Source: CAD feature listing. Evaluate the final solid. Frame: model axes, mm. Face numbers are marked on the shaded views. Give positions to 0.01 mm unless a question says otherwise; leave off trailing zeros. Write each loop counter-clockwise with the first axis right and the second up, starting at its lowest first coordinate (ties: lowest second). Pieces come first, ordered by that corner, then holes. Notation, with made-up numbers: M 41.25,68 L 83.25,68 A23 ccw 83.25,86 Z; hole C 40.5,31 d11. An arc over 180 degrees is marked long. Return JSON: item names as keys, results as strings.
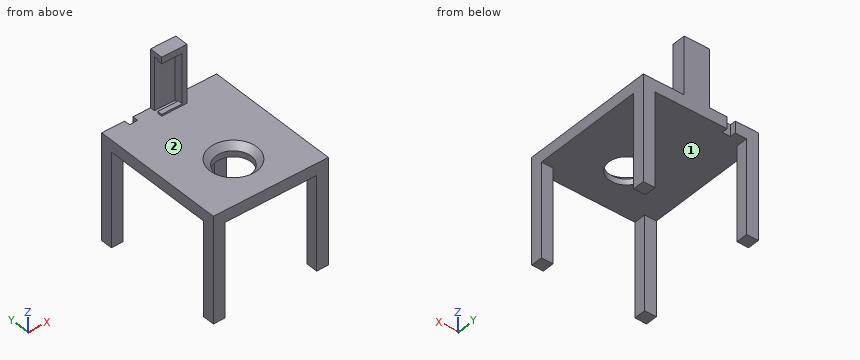
Autodesk Inventor part; units mm, degrees
ref_plane "YZ Plane" through (0, 0, 0) normal (1, 0, 0) x (0, 1, 0)
ref_plane "XZ Plane" through (0, 0, 0) normal (0, 1, 0) x (-1, 0, 0)
ref_plane "XY Plane" through (0, 0, 0) normal (0, 0, 1) x (1, 0, 0)
sketch "Skizze1" plane through (0, 0, 0) normal (0, 0, 1) x (1, 0, 0)
  line L0 (-19.6, 0) -> (117.6, 0)
  line L1 (0, -23) -> (0, 138)
  line L2 (0, 0) -> (98, 0)
  line L3 (98, 0) -> (98, 115)
  line L4 (98, 115) -> (0, 115)
  line L5 (0, 115) -> (0, 0)
  point P0 (0, 115)
  dimension "d0" = 115
  dimension "d1" = 98
extrude "Extrusion1" add sketch "Skizze1" along normal blind 10
sketch "Skizze2" plane through (0, 0, 10) normal (0, 0, 1) x (1, 0, 0)
  line L0 (98, 115) -> (0, 115)
  line L1 (41.65, 115) -> (63.15, 115)
  line L2 (63.15, 115) -> (63.15, 103.5)
  line L3 (63.15, 103.5) -> (41.65, 103.5)
  line L4 (41.65, 103.5) -> (41.65, 115)
  line L5 (98, 0) -> (98, 115)
  point P0 (0, 0)
  dimension "d4" = 21.5
  dimension "d5" = 11.5
  dimension "d6" = 34.85
extrude "Extrusion2" add sketch "Skizze2" along normal blind 49.2
sketch "Skizze3" plane through (41.65, 103.5, 10) normal (-1, 0, 0) x (0, 0, 1)
  line L0 (45.2, 7.5) -> (45.2, 4)
  line L1 (45.2, 4) -> (43.7, 4)
  line L2 (43.7, 4) -> (43.7, 2.8888)
  line L3 (0, 0) -> (0, 11.5)
  line L4 (45.2, 7.5) -> (0, 7.5)
  line L5 (0, 11.5) -> (0, 0)
  line L6 (0, 4) -> (0, 7.5)
  line L7 (49.2, 11.5) -> (49.2, 0)
  line L8 (0, 11.5) -> (49.2, 11.5)
  line L9 (0, 0) -> (49.2, 0)
  line L10 (1.5, 2.8888) -> (1.5, 4)
  line L11 (1.5, 4) -> (0, 4)
  line L12 (43.7, 2.8888) -> (43.7, 0)
  line L13 (1.5, 2.8888) -> (1.5, 0)
  point P0 (-10, -103.5)
  point P1 (0, 4)
  dimension "d9" = 4
  dimension "d10" = 4
  dimension "d11" = 4
  dimension "d12" = 4
  dimension "d13" = 1.5
  dimension "d14" = 1.5
extrude "Extrusion3" cut sketch "Skizze3" against normal blind 17.5 contours L0 L1 L2 L12 L9 L13 L10 L11 L3 L4
sketch "Skizze4" plane through (0, 0, 10) normal (0, 0, 1) x (1, 0, 0)
  line L0 (98, 115) -> (0, 115)
  line L1 (19.65, 115) -> (26.65, 115)
  line L2 (26.65, 115) -> (26.65, 110)
  line L3 (26.65, 110) -> (19.65, 110)
  line L4 (19.65, 110) -> (19.65, 115)
  line L5 (41.65, 115) -> (41.65, 103.5)
  point P0 (0, 0)
  dimension "d17" = 7
  dimension "d18" = 5
  dimension "d19" = 15
extrude "Extrusion4" cut sketch "Skizze4" against normal blind 10
sketch "Skizze5" plane through (0, 0, 0) normal (0, 0, -1) x (-1, 0, 0)
  line L0 (-19.65, 115) -> (0, 115)
  line L1 (0, 115) -> (0, 0)
  line L2 (-10, 115) -> (0, 115)
  line L3 (0, 115) -> (0, 105)
  line L4 (0, 105) -> (-10, 105)
  line L5 (-10, 105) -> (-10, 115)
  line L6 (0, 0) -> (-98, 0)
  line L7 (0, 10) -> (-10, 10)
  line L8 (-10, 10) -> (-10, 0)
  line L9 (-10, 0) -> (0, 0)
  line L10 (0, 0) -> (0, 10)
  line L11 (-98, 10) -> (-88, 10)
  line L12 (-88, 10) -> (-88, 0)
  line L13 (-88, 0) -> (-98, 0)
  line L14 (-98, 0) -> (-98, 10)
  line L15 (-98, 115) -> (-26.65, 115)
  line L16 (-88, 115) -> (-98, 115)
  line L17 (-98, 115) -> (-98, 105)
  line L18 (-98, 105) -> (-88, 105)
  line L19 (-88, 105) -> (-88, 115)
  line L20 (-98, 0) -> (-98, 115)
  point P0 (-98, 0)
  point P1 (-88, 0)
  dimension "d22" = 10
  dimension "d23" = 10
  dimension "d24" = 10
  dimension "d25" = 10
  dimension "d26" = 10
  dimension "d27" = 10
  dimension "d28" = 10
  dimension "d29" = 10
  dimension "d40" = 0
extrude "Extrusion5" add sketch "Skizze5" along normal blind 80
sketch "Skizze6" plane through (0, 0, 10) normal (0, 0, 1) x (1, 0, 0)
  circle A0 centre (49, 38.5) radius 15
  line L0 (0, 115) -> (0, 0)
  line L1 (41.65, 103.5) -> (63.15, 103.5)
  dimension "d32" = 30
  dimension "d33" = 49
  dimension "d34" = 65
extrude "Extrusion6" cut sketch "Skizze6" against normal blind 10
chamfer "Fase1" distance 5 angle 45 1 edges at (34, 38.5, 10)
properties part number "Senso_Halter" material "Acetalharz, Schwarz"
1) Cut plane C-C, the plane y = 38.5. Return the cut outline in (x, z), then the cut area to 3 significant figures.
Numbers:
{"outline": "M 0,0 L 34,0 L 34,5 L 29,10 L 0,10 Z; M 64,0 L 98,0 L 98,10 L 69,10 L 64,5 Z", "area": "655 mm²"}
2) Cut plane A-A, the plane x = 49. Return the cut outline in (y, z).
Numbers:
{"outline": "M 0,0 L 23.5,0 L 23.5,5 L 18.5,10 L 0,10 Z; M 53.5,0 L 115,0 L 115,59.2 L 103.5,59.2 L 103.5,53.7 L 107.5,53.7 L 107.5,55.2 L 111,55.2 L 111,10 L 107.5,10 L 107.5,11.5 L 103.5,11.5 L 103.5,10 L 58.5,10 L 53.5,5 Z"}
3) Draft query along X for the marked faces 1 and 2. Return one class per face: released by +X, released by -X, zero draft, split by the parting line, or undercut.
Numbers:
{"face 1": "undercut", "face 2": "zero draft"}
4) Contact query for flat-ended pins moving along their axis: pin 1 Ø12.5 at (y, z) = (111.5, 32) entering from -X; pin 2 Ø5 at (x, z) = (50, 32.5) entering from -Y; pin 3 Ø8 at (x, y) = (71, 63) entering from -Z; pin 4 Ø1.5 at (y, z) = (24.5, 12.5) entering from +X. Output: stop coordinate, or through.
Numbers:
{"pin 1": "stops at x = 41.65", "pin 2": "stops at y = 111", "pin 3": "stops at z = 0", "pin 4": "passes through"}
5) Cut plane B-B, the plane z = -62. Return the cut outline in (x, y).
Numbers:
{"outline": "M 0,0 L 10,0 L 10,10 L 0,10 Z; M 0,105 L 10,105 L 10,115 L 0,115 Z; M 88,0 L 98,0 L 98,10 L 88,10 Z; M 88,105 L 98,105 L 98,115 L 88,115 Z"}
6) Cut plane D-D, the plane x = 91. Return the cut outline in (y, z), then the cut area to 3 significant figures.
Numbers:
{"outline": "M 0,-80 L 10,-80 L 10,0 L 105,0 L 105,-80 L 115,-80 L 115,10 L 0,10 Z", "area": "2,750 mm²"}
7) Line query: line 1 (Y direction, x = 49, z = 3.4); line 2 (Y direction, x = 51, z = 10.5); line 3 (Z direction, x = 84.5, y = 12.5). Output: solid intervals per line, ascending. Write a range as [from, to].
Numbers:
{"line 1": "y = [0, 23.5], [53.5, 115]", "line 2": "y = [103.5, 107.5], [111, 115]", "line 3": "z = [0, 10]"}
